Build history of the part. All positions in model axes, mm. Face numbers are marked on the shaded views. Coordinates: 2 decimals unless noted, no trailing zeros. Loops run counter-clockwise (first coordinate to the right, second up) from the corner with the lowest first, then second, coordinate; pieces in that order, holes last.
Item 1: Drill centre lines: line 1 along Z through (x, y) = (0.5, -9); line 2 along X through (y, z) = (-8.75, 9.25); line 3 along X through (y, z) = (-4, 1.75). Where is each one in solid material? Low to high.
Item 2: Flat gauge pins, fed straight in: pin 1 (1 mm diameter, centred on x = 43.5, z = 4.5, fed in from -Y); pin 2 (1 mm diameter, centred on y = -3.5, z = 14, fed in from +X); pin 3 (4 mm diameter, centred on y = -10.5, z = 14.5, fed in from -X). Where does each tip first touch, or does it go through?
Item 3: Mould opens along X. For the marked faces 1, 2 and 3 say: released by +X, released by -X, zero draft, split by the parting line, or undercut.
Item 4: Cut at A-A (y = -9.5). List the corners of the cut face in (x, z), and give its area (3 significant figures).
from build123d import *

# Parameters (mm, degrees)
PAD_DEPTH   = 20
FILLET_R    = 4
FILLET001_R = 4
FILLET002_R = 3
FILLET003_R = 3


with BuildPart() as part:
    # Sketch → Pad (new body)
    with BuildSketch(Plane.XZ):
        with BuildLine():
            ThreePointArc((50, 0), (0, 17.55002), (-50, 0))
            Line((-70, 0), (-50, 0))
            ThreePointArc((70, 0), (0, 25.147186), (-70, 0))
            Line((50, 0), (70, 0))
        make_face()
    extrude(amount=PAD_DEPTH)

    # Fillet
    fillet_edges = [part.edges().sort_by_distance(p)[0] for p in [
        (0, -20, 25.147186),
    ]]
    fillet(fillet_edges, radius=FILLET_R)

    # Fillet001
    fillet001_edges = [part.edges().sort_by_distance(p)[0] for p in [
        (0, 0, 25.147186),
    ]]
    fillet(fillet001_edges, radius=FILLET001_R)

    # Fillet002
    fillet002_edges = [part.edges().sort_by_distance(p)[0] for p in [
        (0, 0, 17.55002),
    ]]
    fillet(fillet002_edges, radius=FILLET002_R)

    # Fillet003
    fillet003_edges = [part.edges().sort_by_distance(p)[0] for p in [
        (0, -20, 17.55002),
    ]]
    fillet(fillet003_edges, radius=FILLET003_R)


solid = part.part
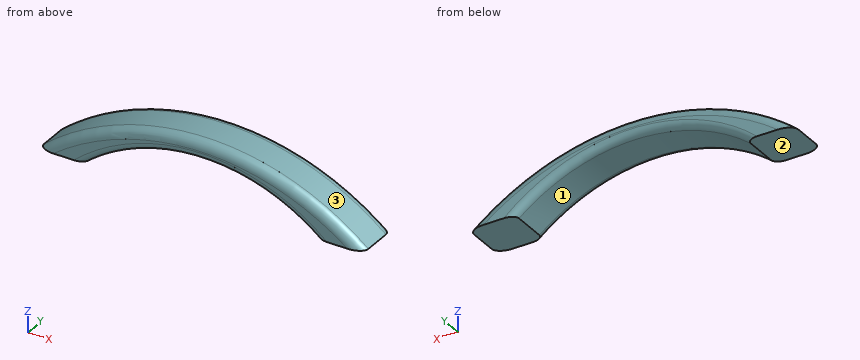
Filled sheet:
1. line 1: z = 17.55 to 25.15
1. line 2: x = -56.96 to -35.48, 35.48 to 56.96
1. line 3: x = -67.82 to -47.73, 47.73 to 67.82
2. pin 1: stops at y = -18.39
2. pin 2: stops at x = 49.2
2. pin 3: stops at x = -51.21
3. face 1: undercut
3. face 2: zero draft
3. face 3: split by the parting line
4. outline: (-70, 0) - (-50, 0) arc R80 cw to (50, 0) - (70, 0) arc R110 ccw to start
4. area: 1,210 mm2
